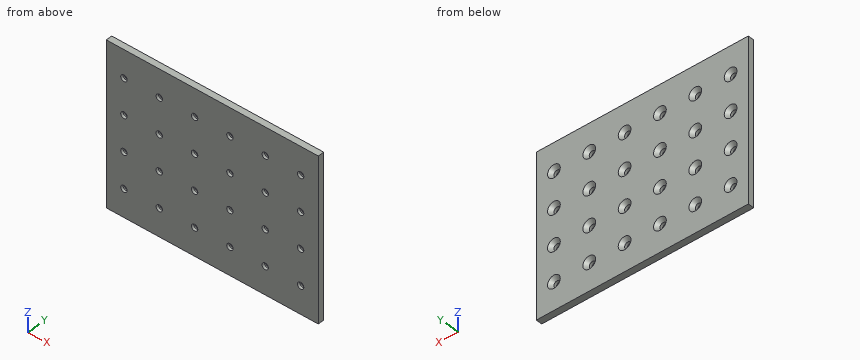
from build123d import *

# Parameters (mm, degrees)
SKETCH1_W                                     = 108
SKETCH1_H                                     = 82
SKETCH1_R                                     = 1.63195
BOSS_EXTRUDE1_DEPTH                           = 3.175
CSK_FOR_4_FLAT_HEAD_MACHINE_SCREW1_AT_2_COUNT = 2
CSK_FOR_4_FLAT_HEAD_MACHINE_SCREW1_AT_2_PITCH = 18
CSK_FOR_4_FLAT_HEAD_MACHINE_SCREW1_AT_3_COUNT = 2
CSK_FOR_4_FLAT_HEAD_MACHINE_SCREW1_AT_3_PITCH = 36
CSK_FOR_4_FLAT_HEAD_MACHINE_SCREW1_AT_4_COUNT = 2
CSK_FOR_4_FLAT_HEAD_MACHINE_SCREW1_AT_4_PITCH = 54
CSK_FOR_4_FLAT_HEAD_MACHINE_SCREW1_AT_5_COUNT = 2
CSK_FOR_4_FLAT_HEAD_MACHINE_SCREW1_AT_5_PITCH = 72
CSK_FOR_4_FLAT_HEAD_MACHINE_SCREW1_AT_6_COUNT = 2
CSK_FOR_4_FLAT_HEAD_MACHINE_SCREW1_AT_6_PITCH = 90
CSK_FOR_4_FLAT_HEAD_MACHINE_SCREW1_AT_7_COUNT = 2
CSK_FOR_4_FLAT_HEAD_MACHINE_SCREW1_AT_7_PITCH = 91.782351245
CSK_FOR_4_FLAT_HEAD_MACHINE_SCREW1_AT_8_COUNT = 2
CSK_FOR_4_FLAT_HEAD_MACHINE_SCREW1_AT_8_PITCH = 74.215901261
CSK_FOR_4_FLAT_HEAD_MACHINE_SCREW1_AT_9_COUNT = 2
CSK_FOR_4_FLAT_HEAD_MACHINE_SCREW1_AT_9_PITCH = 56.920997883
CSK_FOR_4_FLAT_HEAD_MACHINE_SCREW1_AT_1_COUNT = 2
CSK_FOR_4_FLAT_HEAD_MACHINE_SCREW1_AT_1_PITCH = 40.249223595
CSK_FOR_4_FLAT_HEAD_MACHINE_SCREW1_2_COUNT    = 2
CSK_FOR_4_FLAT_HEAD_MACHINE_SCREW1_2_PITCH    = 25.455844123
CSK_FOR_4_FLAT_HEAD_MACHINE_SCREW1_3_COUNT    = 2
CSK_FOR_4_FLAT_HEAD_MACHINE_SCREW1_3_PITCH    = 18
CSK_FOR_4_FLAT_HEAD_MACHINE_SCREW1_4_COUNT    = 2
CSK_FOR_4_FLAT_HEAD_MACHINE_SCREW1_4_PITCH    = 36
CSK_FOR_4_FLAT_HEAD_MACHINE_SCREW1_5_COUNT    = 2
CSK_FOR_4_FLAT_HEAD_MACHINE_SCREW1_5_PITCH    = 40.249223595
CSK_FOR_4_FLAT_HEAD_MACHINE_SCREW1_6_COUNT    = 2
CSK_FOR_4_FLAT_HEAD_MACHINE_SCREW1_6_PITCH    = 50.911688245
CSK_FOR_4_FLAT_HEAD_MACHINE_SCREW1_7_COUNT    = 2
CSK_FOR_4_FLAT_HEAD_MACHINE_SCREW1_7_PITCH    = 64.899922958
CSK_FOR_4_FLAT_HEAD_MACHINE_SCREW1_8_COUNT    = 2
CSK_FOR_4_FLAT_HEAD_MACHINE_SCREW1_8_PITCH    = 80.49844719
CSK_FOR_4_FLAT_HEAD_MACHINE_SCREW1_9_COUNT    = 2
CSK_FOR_4_FLAT_HEAD_MACHINE_SCREW1_9_PITCH    = 96.932966528
CSK_FOR_4_FLAT_HEAD_MACHINE_SCREW1_10_COUNT   = 2
CSK_FOR_4_FLAT_HEAD_MACHINE_SCREW1_10_PITCH   = 104.957134107
CSK_FOR_4_FLAT_HEAD_MACHINE_SCREW1_11_COUNT   = 2
CSK_FOR_4_FLAT_HEAD_MACHINE_SCREW1_11_PITCH   = 90
CSK_FOR_4_FLAT_HEAD_MACHINE_SCREW1_12_COUNT   = 2
CSK_FOR_4_FLAT_HEAD_MACHINE_SCREW1_12_PITCH   = 76.367532368
CSK_FOR_4_FLAT_HEAD_MACHINE_SCREW1_13_COUNT   = 2
CSK_FOR_4_FLAT_HEAD_MACHINE_SCREW1_13_PITCH   = 64.899922958
CSK_FOR_4_FLAT_HEAD_MACHINE_SCREW1_14_COUNT   = 2
CSK_FOR_4_FLAT_HEAD_MACHINE_SCREW1_14_PITCH   = 56.920997883
CSK_FOR_4_FLAT_HEAD_MACHINE_SCREW1_15_COUNT   = 2
CSK_FOR_4_FLAT_HEAD_MACHINE_SCREW1_15_PITCH   = 54


with BuildPart() as part:
    # Sketch1 → Boss-Extrude1 (new body)
    with BuildSketch(Plane(origin=(0, 0, 0), x_dir=(1, 0, 0), z_dir=(0, 1, 0))):
        Rectangle(SKETCH1_W, SKETCH1_H)
        with Locations(Location((-45, 27, 0), (0, 0, 270))):
            Circle(SKETCH1_R, mode=Mode.SUBTRACT)
        with Locations(Location((-27, 27, 0), (0, 0, 270))):
            Circle(SKETCH1_R, mode=Mode.SUBTRACT)
        with Locations(Location((-9, 27, 0), (0, 0, 270))):
            Circle(SKETCH1_R, mode=Mode.SUBTRACT)
        with Locations(Location((9, 27, 0), (0, 0, 270))):
            Circle(SKETCH1_R, mode=Mode.SUBTRACT)
        with Locations(Location((27, 27, 0), (0, 0, 270))):
            Circle(SKETCH1_R, mode=Mode.SUBTRACT)
        with Locations(Location((45, 27, 0), (0, 0, 270))):
            Circle(SKETCH1_R, mode=Mode.SUBTRACT)
        with Locations(Location((-27, 9, 0), (0, 0, 270))):
            Circle(SKETCH1_R, mode=Mode.SUBTRACT)
        with Locations(Location((-9, 9, 0), (0, 0, 270))):
            Circle(SKETCH1_R, mode=Mode.SUBTRACT)
        with Locations(Location((9, 9, 0), (0, 0, 270))):
            Circle(SKETCH1_R, mode=Mode.SUBTRACT)
        with Locations(Location((27, 9, 0), (0, 0, 270))):
            Circle(SKETCH1_R, mode=Mode.SUBTRACT)
        with Locations(Location((45, 9, 0), (0, 0, 270))):
            Circle(SKETCH1_R, mode=Mode.SUBTRACT)
        with Locations(Location((-27, -9, 0), (0, 0, 270))):
            Circle(SKETCH1_R, mode=Mode.SUBTRACT)
        with Locations(Location((-9, -9, 0), (0, 0, 270))):
            Circle(SKETCH1_R, mode=Mode.SUBTRACT)
        with Locations(Location((9, -9, 0), (0, 0, 270))):
            Circle(SKETCH1_R, mode=Mode.SUBTRACT)
        with Locations(Location((27, -9, 0), (0, 0, 270))):
            Circle(SKETCH1_R, mode=Mode.SUBTRACT)
        with Locations(Location((45, -9, 0), (0, 0, 270))):
            Circle(SKETCH1_R, mode=Mode.SUBTRACT)
        with Locations(Location((-27, -27, 0), (0, 0, 270))):
            Circle(SKETCH1_R, mode=Mode.SUBTRACT)
        with Locations(Location((-9, -27, 0), (0, 0, 270))):
            Circle(SKETCH1_R, mode=Mode.SUBTRACT)
        with Locations(Location((9, -27, 0), (0, 0, 270))):
            Circle(SKETCH1_R, mode=Mode.SUBTRACT)
        with Locations(Location((27, -27, 0), (0, 0, 270))):
            Circle(SKETCH1_R, mode=Mode.SUBTRACT)
        with Locations(Location((45, -27, 0), (0, 0, 270))):
            Circle(SKETCH1_R, mode=Mode.SUBTRACT)
        with Locations(Location((-45, 9, 0), (0, 0, 270))):
            Circle(SKETCH1_R, mode=Mode.SUBTRACT)
        with Locations(Location((-45, -9, 0), (0, 0, 270))):
            Circle(SKETCH1_R, mode=Mode.SUBTRACT)
        with Locations(Location((-45, -27, 0), (0, 0, 270))):
            Circle(SKETCH1_R, mode=Mode.SUBTRACT)
    extrude(amount=BOSS_EXTRUDE1_DEPTH)

    # Sketch3 → CSK for #4 Flat Head Machine Screw1 (revolve, cut)
    with BuildSketch(Plane(origin=(45, 3.175, 27), x_dir=(0, 0, 1), z_dir=(1, 0, 0))):
        Polygon((0, 0), (0, 3.175), (1.63195, 3.175), (1.63195, 1.848124365), (3.2385, 0), align=None)
    csk_for_4_flat_head_machine_screw1 = revolve(axis=Axis((45, 9.525, 27), (0, -1, 0)), mode=Mode.SUBTRACT)

    # CSK for #4 Flat Head Machine Screw1 at 2: CSK for #4 Flat Head Machine Screw1 ×2
    with Locations(*[(-i * CSK_FOR_4_FLAT_HEAD_MACHINE_SCREW1_AT_2_PITCH, 0, 0) for i in range(1, CSK_FOR_4_FLAT_HEAD_MACHINE_SCREW1_AT_2_COUNT)]):
        add(csk_for_4_flat_head_machine_screw1, mode=Mode.SUBTRACT)

    # CSK for #4 Flat Head Machine Screw1 at 3: CSK for #4 Flat Head Machine Screw1 ×2
    with Locations(*[(-i * CSK_FOR_4_FLAT_HEAD_MACHINE_SCREW1_AT_3_PITCH, 0, 0) for i in range(1, CSK_FOR_4_FLAT_HEAD_MACHINE_SCREW1_AT_3_COUNT)]):
        add(csk_for_4_flat_head_machine_screw1, mode=Mode.SUBTRACT)

    # CSK for #4 Flat Head Machine Screw1 at 4: CSK for #4 Flat Head Machine Screw1 ×2
    with Locations(*[(-i * CSK_FOR_4_FLAT_HEAD_MACHINE_SCREW1_AT_4_PITCH, 0, 0) for i in range(1, CSK_FOR_4_FLAT_HEAD_MACHINE_SCREW1_AT_4_COUNT)]):
        add(csk_for_4_flat_head_machine_screw1, mode=Mode.SUBTRACT)

    # CSK for #4 Flat Head Machine Screw1 at 5: CSK for #4 Flat Head Machine Screw1 ×2
    with Locations(*[(-i * CSK_FOR_4_FLAT_HEAD_MACHINE_SCREW1_AT_5_PITCH, 0, 0) for i in range(1, CSK_FOR_4_FLAT_HEAD_MACHINE_SCREW1_AT_5_COUNT)]):
        add(csk_for_4_flat_head_machine_screw1, mode=Mode.SUBTRACT)

    # CSK for #4 Flat Head Machine Screw1 at 6: CSK for #4 Flat Head Machine Screw1 ×2
    with Locations(*[(-i * CSK_FOR_4_FLAT_HEAD_MACHINE_SCREW1_AT_6_PITCH, 0, 0) for i in range(1, CSK_FOR_4_FLAT_HEAD_MACHINE_SCREW1_AT_6_COUNT)]):
        add(csk_for_4_flat_head_machine_screw1, mode=Mode.SUBTRACT)

    # CSK for #4 Flat Head Machine Screw1 at 7: CSK for #4 Flat Head Machine Screw1 ×2
    with Locations(*[Vector(-0.9805806756909203, 0, -0.1961161351381836) * (i * CSK_FOR_4_FLAT_HEAD_MACHINE_SCREW1_AT_7_PITCH) for i in range(1, CSK_FOR_4_FLAT_HEAD_MACHINE_SCREW1_AT_7_COUNT)]):
        add(csk_for_4_flat_head_machine_screw1, mode=Mode.SUBTRACT)

    # CSK for #4 Flat Head Machine Screw1 at 8: CSK for #4 Flat Head Machine Screw1 ×2
    with Locations(*[Vector(-0.9701425001453321, 0, -0.24253562503633236) * (i * CSK_FOR_4_FLAT_HEAD_MACHINE_SCREW1_AT_8_PITCH) for i in range(1, CSK_FOR_4_FLAT_HEAD_MACHINE_SCREW1_AT_8_COUNT)]):
        add(csk_for_4_flat_head_machine_screw1, mode=Mode.SUBTRACT)

    # CSK for #4 Flat Head Machine Screw1 at 9: CSK for #4 Flat Head Machine Screw1 ×2
    with Locations(*[Vector(-0.9486832980505142, 0, -0.31622776601683683) * (i * CSK_FOR_4_FLAT_HEAD_MACHINE_SCREW1_AT_9_PITCH) for i in range(1, CSK_FOR_4_FLAT_HEAD_MACHINE_SCREW1_AT_9_COUNT)]):
        add(csk_for_4_flat_head_machine_screw1, mode=Mode.SUBTRACT)

    # CSK for #4 Flat Head Machine Screw1 at 1: CSK for #4 Flat Head Machine Screw1 ×2
    with Locations(*[Vector(-0.894427190999917, 0, -0.44721359549995593) * (i * CSK_FOR_4_FLAT_HEAD_MACHINE_SCREW1_AT_1_PITCH) for i in range(1, CSK_FOR_4_FLAT_HEAD_MACHINE_SCREW1_AT_1_COUNT)]):
        add(csk_for_4_flat_head_machine_screw1, mode=Mode.SUBTRACT)

    # CSK for #4 Flat Head Machine Screw1  2: CSK for #4 Flat Head Machine Screw1 ×2
    with Locations(*[Vector(-0.7071067811865515, 0, -0.7071067811865436) * (i * CSK_FOR_4_FLAT_HEAD_MACHINE_SCREW1_2_PITCH) for i in range(1, CSK_FOR_4_FLAT_HEAD_MACHINE_SCREW1_2_COUNT)]):
        add(csk_for_4_flat_head_machine_screw1, mode=Mode.SUBTRACT)

    # CSK for #4 Flat Head Machine Screw1  3: CSK for #4 Flat Head Machine Screw1 ×2
    with Locations(*[(0, 0, -i * CSK_FOR_4_FLAT_HEAD_MACHINE_SCREW1_3_PITCH) for i in range(1, CSK_FOR_4_FLAT_HEAD_MACHINE_SCREW1_3_COUNT)]):
        add(csk_for_4_flat_head_machine_screw1, mode=Mode.SUBTRACT)

    # CSK for #4 Flat Head Machine Screw1  4: CSK for #4 Flat Head Machine Screw1 ×2
    with Locations(*[(0, 0, -i * CSK_FOR_4_FLAT_HEAD_MACHINE_SCREW1_4_PITCH) for i in range(1, CSK_FOR_4_FLAT_HEAD_MACHINE_SCREW1_4_COUNT)]):
        add(csk_for_4_flat_head_machine_screw1, mode=Mode.SUBTRACT)

    # CSK for #4 Flat Head Machine Screw1  5: CSK for #4 Flat Head Machine Screw1 ×2
    with Locations(*[Vector(-0.44721359549996553, 0, -0.8944271909999122) * (i * CSK_FOR_4_FLAT_HEAD_MACHINE_SCREW1_5_PITCH) for i in range(1, CSK_FOR_4_FLAT_HEAD_MACHINE_SCREW1_5_COUNT)]):
        add(csk_for_4_flat_head_machine_screw1, mode=Mode.SUBTRACT)

    # CSK for #4 Flat Head Machine Screw1  6: CSK for #4 Flat Head Machine Screw1 ×2
    with Locations(*[Vector(-0.7071067811865513, 0, -0.7071067811865437) * (i * CSK_FOR_4_FLAT_HEAD_MACHINE_SCREW1_6_PITCH) for i in range(1, CSK_FOR_4_FLAT_HEAD_MACHINE_SCREW1_6_COUNT)]):
        add(csk_for_4_flat_head_machine_screw1, mode=Mode.SUBTRACT)

    # CSK for #4 Flat Head Machine Screw1  7: CSK for #4 Flat Head Machine Screw1 ×2
    with Locations(*[Vector(-0.8320502943378456, 0, -0.5547001962252264) * (i * CSK_FOR_4_FLAT_HEAD_MACHINE_SCREW1_7_PITCH) for i in range(1, CSK_FOR_4_FLAT_HEAD_MACHINE_SCREW1_7_COUNT)]):
        add(csk_for_4_flat_head_machine_screw1, mode=Mode.SUBTRACT)

    # CSK for #4 Flat Head Machine Screw1  8: CSK for #4 Flat Head Machine Screw1 ×2
    with Locations(*[Vector(-0.894427190999917, 0, -0.447213595499956) * (i * CSK_FOR_4_FLAT_HEAD_MACHINE_SCREW1_8_PITCH) for i in range(1, CSK_FOR_4_FLAT_HEAD_MACHINE_SCREW1_8_COUNT)]):
        add(csk_for_4_flat_head_machine_screw1, mode=Mode.SUBTRACT)

    # CSK for #4 Flat Head Machine Screw1  9: CSK for #4 Flat Head Machine Screw1 ×2
    with Locations(*[Vector(-0.9284766908852599, 0, -0.37139067635410233) * (i * CSK_FOR_4_FLAT_HEAD_MACHINE_SCREW1_9_PITCH) for i in range(1, CSK_FOR_4_FLAT_HEAD_MACHINE_SCREW1_9_COUNT)]):
        add(csk_for_4_flat_head_machine_screw1, mode=Mode.SUBTRACT)

    # CSK for #4 Flat Head Machine Screw1  10: CSK for #4 Flat Head Machine Screw1 ×2
    with Locations(*[Vector(-0.8574929257125457, 0, -0.514495755427524) * (i * CSK_FOR_4_FLAT_HEAD_MACHINE_SCREW1_10_PITCH) for i in range(1, CSK_FOR_4_FLAT_HEAD_MACHINE_SCREW1_10_COUNT)]):
        add(csk_for_4_flat_head_machine_screw1, mode=Mode.SUBTRACT)

    # CSK for #4 Flat Head Machine Screw1  11: CSK for #4 Flat Head Machine Screw1 ×2
    with Locations(*[Vector(-0.8000000000000023, 0, -0.5999999999999969) * (i * CSK_FOR_4_FLAT_HEAD_MACHINE_SCREW1_11_PITCH) for i in range(1, CSK_FOR_4_FLAT_HEAD_MACHINE_SCREW1_11_COUNT)]):
        add(csk_for_4_flat_head_machine_screw1, mode=Mode.SUBTRACT)

    # CSK for #4 Flat Head Machine Screw1  12: CSK for #4 Flat Head Machine Screw1 ×2
    with Locations(*[Vector(-0.7071067811865513, 0, -0.7071067811865438) * (i * CSK_FOR_4_FLAT_HEAD_MACHINE_SCREW1_12_PITCH) for i in range(1, CSK_FOR_4_FLAT_HEAD_MACHINE_SCREW1_12_COUNT)]):
        add(csk_for_4_flat_head_machine_screw1, mode=Mode.SUBTRACT)

    # CSK for #4 Flat Head Machine Screw1  13: CSK for #4 Flat Head Machine Screw1 ×2
    with Locations(*[Vector(-0.5547001962252354, 0, -0.8320502943378396) * (i * CSK_FOR_4_FLAT_HEAD_MACHINE_SCREW1_13_PITCH) for i in range(1, CSK_FOR_4_FLAT_HEAD_MACHINE_SCREW1_13_COUNT)]):
        add(csk_for_4_flat_head_machine_screw1, mode=Mode.SUBTRACT)

    # CSK for #4 Flat Head Machine Screw1  14: CSK for #4 Flat Head Machine Screw1 ×2
    with Locations(*[Vector(-0.31622776601684705, 0, -0.9486832980505108) * (i * CSK_FOR_4_FLAT_HEAD_MACHINE_SCREW1_14_PITCH) for i in range(1, CSK_FOR_4_FLAT_HEAD_MACHINE_SCREW1_14_COUNT)]):
        add(csk_for_4_flat_head_machine_screw1, mode=Mode.SUBTRACT)

    # CSK for #4 Flat Head Machine Screw1  15: CSK for #4 Flat Head Machine Screw1 ×2
    with Locations(*[(0, 0, -i * CSK_FOR_4_FLAT_HEAD_MACHINE_SCREW1_15_PITCH) for i in range(1, CSK_FOR_4_FLAT_HEAD_MACHINE_SCREW1_15_COUNT)]):
        add(csk_for_4_flat_head_machine_screw1, mode=Mode.SUBTRACT)


solid = part.part
Model file for the job. Use its own axes, mm. Round coordinates to 2 decimals unless told otherwise and drop trailing zeros. Loops run counter-clockwise (first coordinate to the right, second up) from the corner with the lowest first, then second, coordinate; pieces in that order, holes last. Notation, with made-up numbers: (14.25, 44) -> (59.25, 44) arc R17 cw to (59.25, 54) -> close; hole circle Ø2 at (81, 88). An arc over 180 degrees is marked (long way). Answer as CSV lines item,"result". Start each with the question number.
1) Pin check, flat tips, straight feed: P1, Ø5, axis at x = -27, z = 27, coming from the +Y side; P2, Ø2, axis at x = 45, z = 9, coming from the -Y side; P3, Ø4, axis at x = 9, z = -9, coming from the +Y side. Stop position of each tip, or through.
2) Slice it at A-A (y = 0.75). State how many separate pieces and enclosed holes the cut face has, plus the area to 3 significant figures.
3) Slice it at B-B (x = 27). List the corners of the cut face in (y, z) (1 decimal), plus the area to 3 significant figures.
4) Probe line 1 along Z through (x, y) = (-10, 1.35); line 2 along Z through (x, y) = (-46, 1.8). List the from-to ranges inside material, lowest first.
Filled in:
1,P1,"stops at y = 2.33"
1,P2,"passes through"
1,P3,"stops at y = 1.75"
2,separate pieces,"1"
2,enclosed holes,"24"
2,area,"8,660 mm2"
3,outline,"(0, -41) -> (3.2, -41) -> (3.2, -30.2) -> (1.3, -28.6) -> (0, -28.6) -> close; (0, -25.4) -> (1.3, -25.4) -> (3.2, -23.8) -> (3.2, -12.2) -> (1.3, -10.6) -> (0, -10.6) -> close; (0, -7.4) -> (1.3, -7.4) -> (3.2, -5.8) -> (3.2, 5.8) -> (1.3, 7.4) -> (0, 7.4) -> close; (0, 10.6) -> (1.3, 10.6) -> (3.2, 12.2) -> (3.2, 23.8) -> (1.3, 25.4) -> (0, 25.4) -> close; (0, 28.6) -> (1.3, 28.6) -> (3.2, 30.2) -> (3.2, 41) -> (0, 41) -> close"
3,area,"207 mm2"
4,line 1,"z = -41 to -28.32, -25.68 to -10.32, -7.68 to 7.68, 10.32 to 25.68, 28.32 to 41"
4,line 2,"z = -41 to -28.78, -25.22 to -10.78, -7.22 to 7.22, 10.78 to 25.22, 28.78 to 41"
